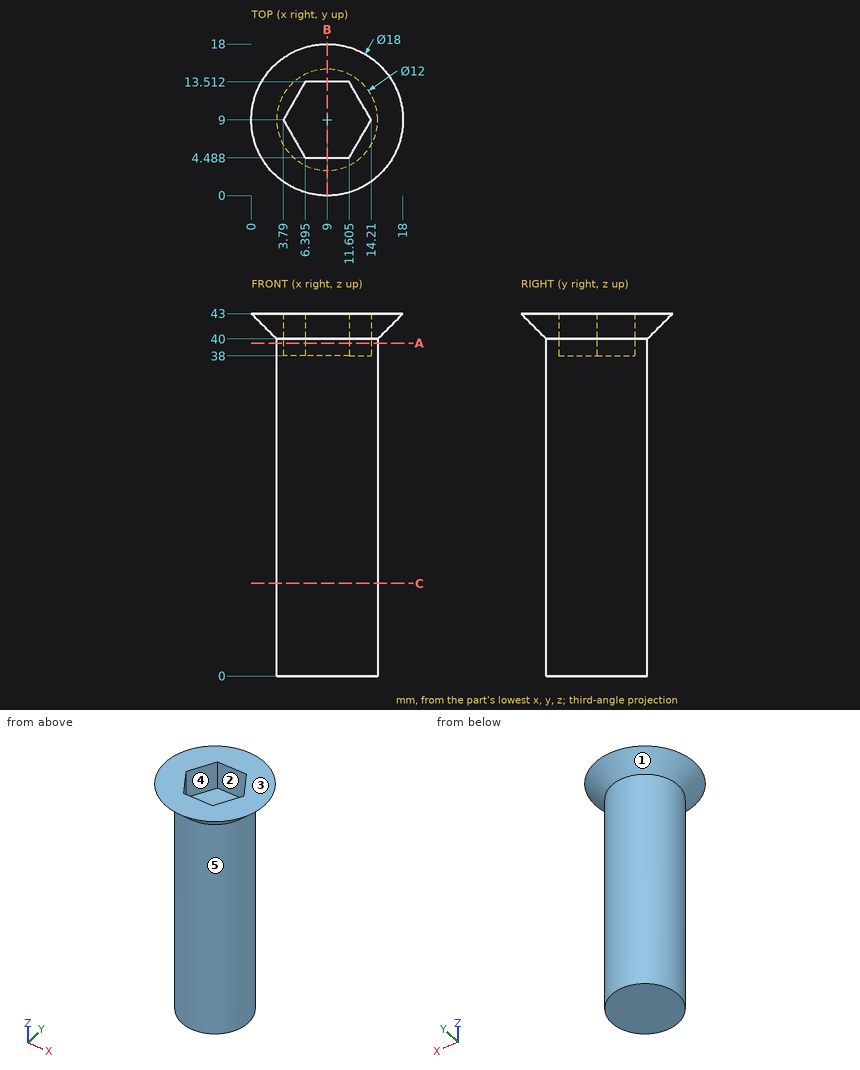
Could you check a few things on this drawing? It's one solid part, dimensions in mm from its lowest x, y, z. A direction names the side the tool comes from. Give positions to 0.01 mm unless a question says otherwise; leave off trailing zeros. Order: outer loops, then holes, each group sorted by start corner. A loop starts at its lowest first (then second) coordinate and runs counter-clockwise, first axis right, second up. Notation, with made-up numbers: M 60.25,10 L 95.25,10 A25 cw 95.25,35 Z; hole C 85,9 d1. An arc over 180 degrees is marked long. Use one line per item in the form item = value. Start each with the question number.
Item 1: We'd pull the mould along X, two halves only. Please class the marked faces 3, 4 and 5: +X half, -X half, draft (parallel to the pull), parting line (faces both ways), or undercut.
Item 2: If we section it at A-A (z = 39.5): Write out the boundary of the cut face in (x, y) (3 decimals), then the cut area to 3 significant figures.
Item 3: If I drill on line 1 along Z through (x, y) = (11.75, 9.5); line 2 along Y through (x, z) = (5.25, 23); line 3 along X through (y, z) = (4.75, 39.5), over which ranges is the centre line in solid material (lowest first)?
Item 4: Will these pins go through, and if not, where does the flat tip stop? pin 1 Ø2 at (x, y) = (9.5, 11) entering from -Z; pin 2 Ø1 at (x, y) = (10, 10) entering from +Z; pin 3 Ø2.5 at (x, z) = (9.5, 40) entering from -Y; pin 4 Ø8 at (x, z) = (12, 17.5) entering from -Y.
Item 5: For the marked faces 1 and 2, which set-ups out of +Z, -Z, +X, -X, +Y, -Y let a thin tool reach every point of the face, with its end or its side?
Item 6: If we section it at B-B (x = 9): Write out the boundary of the cut face in (y, z), then the cut area to 3 significant figures.
Item 7: If we section it at C-C (z = 11): Write out the boundary of the cut face in (x, y).
Outcome:
q1.face_3 = draft
q1.face_4 = undercut
q1.face_5 = parting line
q2.outline = C 9,9 d12; hole M 3.79,9 L 6.395,4.488 L 11.605,4.488 L 14.21,9 L 11.605,13.512 L 6.395,13.512 Z
q2.area = 42.6 mm2
q3.line_1 = 0 to 38
q3.line_2 = 4.32 to 13.68
q3.line_3 = 4.76 to 6.24, 11.76 to 13.24
q4.pin_1 = 0
q4.pin_2 = 38
q4.pin_3 = 1.76
q4.pin_4 = 3
q5.face_1 = -Z
q5.face_2 = +Z
q6.outline = M 0,43 L 3,40 L 3,0 L 15,0 L 15,40 L 18,43 L 13.51,43 L 13.51,38 L 4.49,38 L 4.49,43 Z
q6.area = 480 mm2
q7.outline = C 9,9 d12
